Autodesk Inventor part; units mm, degrees
ref_plane "YZ Plane" through (0, 0, 0) normal (1, 0, 0) x (0, 1, 0)
ref_plane "XZ Plane" through (0, 0, 0) normal (0, 1, 0) x (-1, 0, 0)
ref_plane "XY Plane" through (0, 0, 0) normal (0, 0, 1) x (1, 0, 0)
sketch "Sketch2" plane through (0, 0, 0) normal (0, 1, 0) x (-1, 0, 0)
  arc A0 (0, -1.5) -> (-1.3365, -0.681) centre (0, 0) ccw
  arc A1 (0, -3) -> (-2.673, -1.362) centre (0, 0) ccw
  line L0 (0, -3) -> (-20, -3)
  line L1 (-20, -3) -> (-20, -1.5)
  line L2 (-20, -1.5) -> (0, -1.5)
  line L3 (-1.3365, -0.681) -> (-2.673, -1.362)
  dimension "d0" = 1.5
  dimension "d1" = 1.5
  dimension "d2" = 20
  dimension "d3" = 3
  dimension "d4" = 27
extrude "Extrusion1" add sketch "Sketch2" along normal blind 304.8
sketch "Sketch3" plane through (20, 0, -3) normal (0, 0, -1) x (-1, 0, 0)
  line L0 (0, 0) -> (20, 0)
  line L1 (23, 30) -> (17, 30)
  line L2 (17, 30) -> (17, 10)
  line L3 (17, 10) -> (23, 10)
  line L4 (23, 10) -> (23, 30)
  line L5 (17, 0) -> (17, 304.8)
  dimension "d7" = 10
  dimension "d8" = 20
  dimension "d9" = 6
extrude "Extrusion2" cut sketch "Sketch3" against normal through all
pattern_linear "Rectangular Pattern1" count 25 spacing 40 along (0, 1, 0) of "Extrusion2"
sketch "Sketch4" plane through (20, 0, -1.5) normal (0, 0, 1) x (1, 0, 0)
  line L0 (-20, 70) -> (-20, 90)
  line L1 (-20, 70) -> (-20, 90)
  line L2 (-20, 70) -> (-20, 90)
  line L3 (-20, 70) -> (-20, 90)
  line L4 (-20, 70) -> (-20, 90)
  line L5 (-20, 70) -> (-20, 90)
  line L6 (-20, 70) -> (-20, 90)
  line L7 (-20, 70) -> (-20, 90)
  line L8 (-20, 270) -> (-20, 290)
  line L9 (-20, 190) -> (-20, 210)
  line L10 (-20, 110) -> (-20, 130)
  line L11 (-20, 30) -> (-20, 50)
  line L12 (0, 0) -> (0, 304.8)
  point P0 (-20, 930)
  point P1 (-20, 910)
  point P2 (-20, 850)
  point P3 (-20, 830)
  point P4 (-20, 770)
  point P5 (-20, 750)
  point P6 (-20, 690)
  point P7 (-20, 670)
  point P8 (-20, 610)
  point P9 (-20, 590)
  point P10 (-20, 530)
  point P11 (-20, 510)
  point P12 (-20, 450)
  point P13 (-20, 430)
  point P14 (-20, 370)
  point P15 (-20, 350)
  point P16 (-8, 40)
  point P17 (-8, 120)
  point P18 (-8, 200)
  point P19 (-8, 280)
  point P20 (-8, 360)
  point P21 (-8, 440)
  point P22 (-8, 520)
  point P23 (-8, 600)
  point P24 (-8, 680)
  point P25 (-8, 760)
  point P26 (-8, 840)
  point P27 (-8, 920)
  point P28 (-20, 40)
  point P29 (-20, 120)
  point P30 (-20, 200)
  point P31 (-20, 280)
  point P32 (-20, 360)
  point P33 (-20, 440)
  point P34 (-20, 520)
  point P35 (-20, 600)
  point P36 (-20, 680)
  point P37 (-20, 760)
  point P38 (-20, 840)
  point P39 (-20, 920)
  dimension "d15" = 8
hole "Hole1" at (12, 40, -1.5) at (12, 120, -1.5) at (12, 200, -1.5) at (12, 280, -1.5) at (12, 360, -1.5) at (12, 440, -1.5) at (12, 520, -1.5) at (12, 600, -1.5) at (12, 680, -1.5) at (12, 760, -1.5) at (12, 840, -1.5) at (12, 920, -1.5) direction (0, 0, -1) diameter 3 end through all countersink diameter 6 countersink angle 90
equation "\"d1\" = d0"
properties part number "SIDE 1" material "Steel, Mild"
Read the model definition and answer for the solid it produces. Units are mm, in the model's axes. A direction names the side the tool comes from. Coordinates: 2 decimals unless noted, no trailing zeros. Write each loop counter-clockwise with the first axis right and the second up, starting at its lowest first coordinate (ties: lowest second). Pieces come first, ordered by that corner, then holes. Notation, with made-up numbers: (76, 43) -> (120, 43) arc R33 cw to (120, 81) -> close; hole circle Ø3 at (69.25, -17). An arc over 180 degrees is marked (long way). Return JSON: item names as keys, results as strings.
1. A cutting plane is placed at B-B (y = 219.5). Determine the outline of the cut face in (x, z), and give its area (3 significant figures).
Found:
{"outline": "(3, -3) -> (20, -3) -> (20, -1.5) -> (3, -1.5) -> close", "area": "25.5 mm2"}
2. A tool of negligible diameter and unlimited length cuts with its end or side. For faces 3 (the face through (-1.3, 90, -1.4)), 4 (the face through (-1.5, 4.9, 2.6)), from which of +Z, -Z, +X, -X, +Y, -Y can it reach the whole face along a straight path? Write none if from no direction.
Found:
{"face 3": "+Z, -Z, -X", "face 4": "+Y, -Y"}
3. Determine the mould class of faces 1 (the face through (-1.5, 159.9, 2.6)), 2 (the face through (1.3, 30, 1.3)) for opening direction Y: pulls with the +Y half, pulls with the -Y half, needs draft (parallel to the pull), parting line crosses it, or undercut.
Found:
{"face 1": "needs draft", "face 2": "undercut"}
4. Find the intervals of material crossed by line 1 along X through (y, z) = (247, -0.05); line 2 along Z through (x, y) = (8.5, 40.5); line 3 along Z through (x, y) = (2, 207), in increasing order. Write a range as from..to.
Found:
{"line 1": "-3..-1.5, 1.5..3", "line 2": "-3..-1.5", "line 3": "-3..-1.5, -1.02..2.24"}
5. A cutting plane is placed at A-A (x = 12). Determine the outline of the cut face in (y, z).
Found:
{"outline": "(0, -3) -> (38.5, -3) -> (37, -1.5) -> (0, -1.5) -> close; (41.5, -3) -> (118.5, -3) -> (117, -1.5) -> (43, -1.5) -> close; (121.5, -3) -> (198.5, -3) -> (197, -1.5) -> (123, -1.5) -> close; (201.5, -3) -> (278.5, -3) -> (277, -1.5) -> (203, -1.5) -> close; (281.5, -3) -> (304.8, -3) -> (304.8, -1.5) -> (283, -1.5) -> close"}
6. Each of these flat-tipped pins is pushed along its axis until it touches: P1, Ø1.8, axis at x = 0.5, z = -1, coming from the -Y side; P2, Ø1.8, axis at x = -1, z = 1, coming from the +Y side; P3, Ø10, axis at x = 11, y = 155, coming from the +Z side; P4, Ø12, axis at x = 6.5, y = 251, coming from the +Z side. Where does it stop, or does it pass through?
Found:
{"P1": "y = 0", "P2": "y = 290", "P3": "z = -1.5", "P4": "z = 2.94"}
